Drawing for the job (mm, zero at the part's lowest x, y, z). Coordinates: 2 decimals unless noted, no trailing zeros. Write each loop counter-clockwise with the first axis right and the second up, starting at its lowest first coordinate (ties: lowest second). Pieces come first, ordered by that corner, then holes. Notation, with made-up numbers: M 55.5,79 L 95.5,79 A11 cw 95.5,85 Z; hole C 56,-37.75 d3. An arc over 180 degrees is marked long. Put each result on its own line as item: value. Start each with the question number.
Q1. Cut at C-C (y = 19). Write the cut outline in (x, z).
Q2. Drill centre lines: line 1 along Z through (x, y) = (579.5, 71.5); line 2 along Z through (x, y) = (566, 64.5); line 3 along Y through (x, z) = (839.5, 22.5). Where is each one in solid material? Low to high.
Q3. Cut at A-A (x = 299.5). Write the cut outline in (y, z).
Q4. Cut at B-B (z = 36.5). Write the cut outline in (x, y), then the cut area to 3 significant figures.
Q5. Drop flat-ended pins along their axis: pin 1 (12 mm diameter, centred on x = 177.5, y = 35, fed in from -Z); pin 2 (6 mm diameter, centred on x = 821, z = 33, fed in from -Y). Give the stop position or say it passes through.
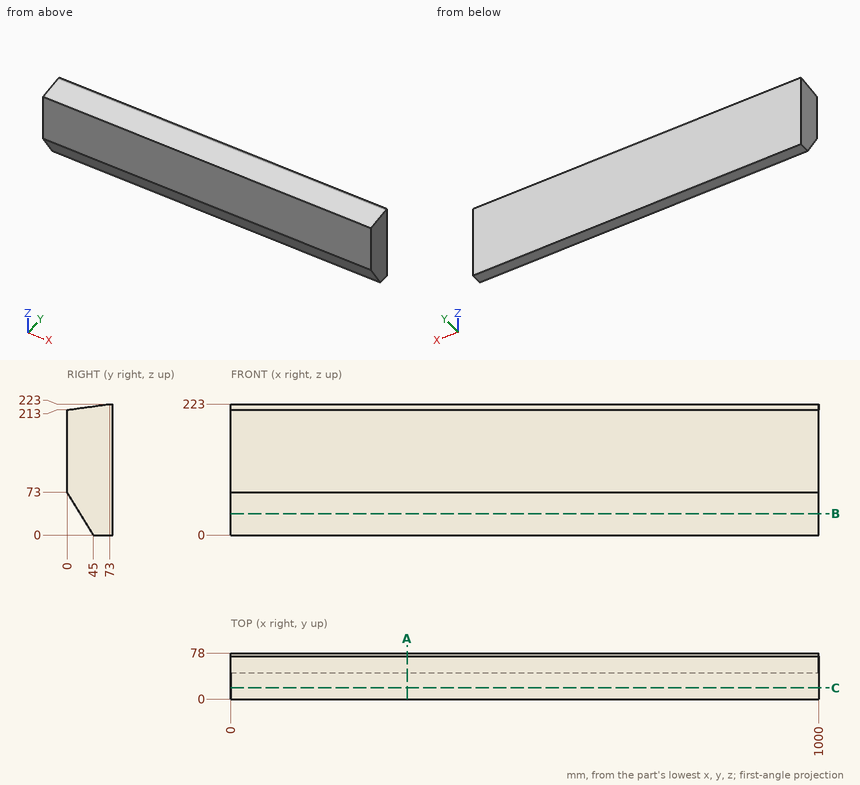
Computed values:
1. outline: M 0,42.18 L 1000,42.18 L 1000,215.6 L 0,215.6 Z
2. line 1: 0 to 222.79
2. line 2: 0 to 221.84
2. line 3: 31.13 to 78
3. outline: M 0,73 L 45,0 L 78,0 L 78,223 L 73,223 L 0,213 Z
4. outline: M 0,22.5 L 1000,22.5 L 1000,78 L 0,78 Z
4. area: 55,500 mm2
5. pin 1: z = 6.49
5. pin 2: y = 22.81
